For this review, take the finished solid that the model builds, in its own axes (mm). A direction names the side the tool comes from. Round coordinates to 2 decimals unless told otherwise and drop trailing zeros. Order: outer loops, then holes, each group sorted by start corner. A loop starts at its lowest first (then second) coordinate and runs counter-clockwise, first axis right, second up. Notation, with made-up numbers: M 3,36 L 16,36 A15 ccw 16,42 Z; hole C 17.5,86.25 d8. An arc over 180 degrees is marked long. Use a Markdown table: item, result.
from build123d import *

# Parameters (mm, degrees)
BOSS_EXTRUDE1_DEPTH = 1
BOSS_EXTRUDE2_START = 1
BOSS_EXTRUDE2_DEPTH = 1.6
BOSS_EXTRUDE3_START = 2.6
BOSS_EXTRUDE3_DEPTH = 1.3
BOSS_EXTRUDE4_START = 3.9
BOSS_EXTRUDE4_DEPTH = 1
FILLET1_R           = 1
CHAMFER1_SIZE       = 1.1


with BuildPart() as part:
    # Sketch1 → Boss-Extrude1 (new body)
    with BuildSketch(Plane(origin=(0, 0, 0), x_dir=(1, 0, 0), z_dir=(0, 1, 0))):
        with BuildLine():
            Line((-18.4, 13.7), (-18.4, 12.505918748))
            ThreePointArc((-18.4, 12.505918748), (-11.9, 4.9), (-18.4, -2.705918748))
            Line((-18.4, -2.705918748), (-18.4, -13.7))
            Line((-18.4, -13.7), (18.4, -13.7))
            Line((18.4, -13.7), (18.4, 13.7))
            Line((18.4, 13.7), (-18.4, 13.7))
        make_face()
        with BuildLine():
            ThreePointArc((-18.4, -2.705918748), (-11.9, 4.9), (-18.4, 12.505918748))
            Line((-18.4, 12.505918748), (-18.4, 10.472252686))
            ThreePointArc((-18.4, 10.472252686), (-13.9, 4.9), (-18.4, -0.672252686))
            Line((-18.4, -0.672252686), (-18.4, -2.705918748))
        make_face()
        with BuildLine():
            Line((19.6, 14.9), (-19.6, 14.9))
            Line((-19.6, 14.9), (-19.6, 12.6))
            ThreePointArc((-19.6, 12.6), (-18.998158808, 12.576443654), (-18.4, 12.505918748))
            Line((-18.4, 12.505918748), (-18.4, 13.7))
            Line((-18.4, 13.7), (18.4, 13.7))
            Line((18.4, 13.7), (18.4, -13.7))
            Line((18.4, -13.7), (-18.4, -13.7))
            Line((-18.4, -13.7), (-18.4, -2.705918748))
            ThreePointArc((-18.4, -2.705918748), (-18.998158808, -2.776443654), (-19.6, -2.8))
            Line((-19.6, -2.8), (-19.6, -14.9))
            Line((-19.6, -14.9), (19.6, -14.9))
            Line((19.6, -14.9), (19.6, 14.9))
        make_face()
        with BuildLine():
            ThreePointArc((-18.4, 12.505918748), (-18.998158808, 12.576443654), (-19.6, 12.6))
            Line((-19.6, 12.6), (-19.6, 10.6))
            ThreePointArc((-19.6, 10.6), (-18.996609708, 10.567973196), (-18.4, 10.472252686))
            Line((-18.4, 10.472252686), (-18.4, 12.505918748))
        make_face()
        with BuildLine():
            ThreePointArc((-18.4, -0.672252686), (-18.996609708, -0.767973196), (-19.6, -0.8))
            Line((-19.6, -0.8), (-19.6, -2.8))
            ThreePointArc((-19.6, -2.8), (-18.998158808, -2.776443654), (-18.4, -2.705918748))
            Line((-18.4, -2.705918748), (-18.4, -0.672252686))
        make_face()
    extrude(amount=BOSS_EXTRUDE1_DEPTH)

    # Sketch1<5> → Boss-Extrude2 (add)
    with BuildSketch(Plane(origin=(0, 0, 0), x_dir=(1, 0, 0), z_dir=(0, 1, 0)).offset(BOSS_EXTRUDE2_START)):
        with BuildLine():
            Line((-18.4, 13.7), (-18.4, 12.505918748))
            ThreePointArc((-18.4, 12.505918748), (-11.9, 4.9), (-18.4, -2.705918748))
            Line((-18.4, -2.705918748), (-18.4, -13.7))
            Line((-18.4, -13.7), (18.4, -13.7))
            Line((18.4, -13.7), (18.4, 13.7))
            Line((18.4, 13.7), (-18.4, 13.7))
        make_face()
        with BuildLine():
            ThreePointArc((-18.4, -2.705918748), (-11.9, 4.9), (-18.4, 12.505918748))
            Line((-18.4, 12.505918748), (-18.4, 10.472252686))
            ThreePointArc((-18.4, 10.472252686), (-13.9, 4.9), (-18.4, -0.672252686))
            Line((-18.4, -0.672252686), (-18.4, -2.705918748))
        make_face()
        with BuildLine():
            ThreePointArc((-18.4, 12.505918748), (-18.998158808, 12.576443654), (-19.6, 12.6))
            Line((-19.6, 12.6), (-19.6, 10.6))
            ThreePointArc((-19.6, 10.6), (-18.996609708, 10.567973196), (-18.4, 10.472252686))
            Line((-18.4, 10.472252686), (-18.4, 12.505918748))
        make_face()
        with BuildLine():
            ThreePointArc((-18.4, -0.672252686), (-18.996609708, -0.767973196), (-19.6, -0.8))
            Line((-19.6, -0.8), (-19.6, -2.8))
            ThreePointArc((-19.6, -2.8), (-18.998158808, -2.776443654), (-18.4, -2.705918748))
            Line((-18.4, -2.705918748), (-18.4, -0.672252686))
        make_face()
        with BuildLine():
            Line((19.6, 14.9), (-19.6, 14.9))
            Line((-19.6, 14.9), (-19.6, 12.6))
            ThreePointArc((-19.6, 12.6), (-18.998158808, 12.576443654), (-18.4, 12.505918748))
            Line((-18.4, 12.505918748), (-18.4, 13.7))
            Line((-18.4, 13.7), (18.4, 13.7))
            Line((18.4, 13.7), (18.4, -13.7))
            Line((18.4, -13.7), (-18.4, -13.7))
            Line((-18.4, -13.7), (-18.4, -2.705918748))
            ThreePointArc((-18.4, -2.705918748), (-18.998158808, -2.776443654), (-19.6, -2.8))
            Line((-19.6, -2.8), (-19.6, -14.9))
            Line((-19.6, -14.9), (19.6, -14.9))
            Line((19.6, -14.9), (19.6, 14.9))
        make_face()
    extrude(amount=BOSS_EXTRUDE2_DEPTH)

    # Sketch1<6> → Boss-Extrude3 (add)
    with BuildSketch(Plane(origin=(0, 0, 0), x_dir=(1, 0, 0), z_dir=(0, 1, 0)).offset(BOSS_EXTRUDE3_START)):
        with BuildLine():
            Line((-18.4, 13.7), (-18.4, 12.505918748))
            ThreePointArc((-18.4, 12.505918748), (-11.9, 4.9), (-18.4, -2.705918748))
            Line((-18.4, -2.705918748), (-18.4, -13.7))
            Line((-18.4, -13.7), (18.4, -13.7))
            Line((18.4, -13.7), (18.4, 13.7))
            Line((18.4, 13.7), (-18.4, 13.7))
        make_face()
        with BuildLine():
            ThreePointArc((-18.4, -2.705918748), (-11.9, 4.9), (-18.4, 12.505918748))
            Line((-18.4, 12.505918748), (-18.4, 10.472252686))
            ThreePointArc((-18.4, 10.472252686), (-13.9, 4.9), (-18.4, -0.672252686))
            Line((-18.4, -0.672252686), (-18.4, -2.705918748))
        make_face()
    extrude(amount=BOSS_EXTRUDE3_DEPTH)

    # Sketch1<8> → Boss-Extrude4 (add)
    with BuildSketch(Plane(origin=(0, 0, 0), x_dir=(1, 0, 0), z_dir=(0, 1, 0)).offset(BOSS_EXTRUDE4_START)):
        with BuildLine():
            ThreePointArc((-18.4, -2.705918748), (-11.9, 4.9), (-18.4, 12.505918748))
            Line((-18.4, 12.505918748), (-18.4, 10.472252686))
            ThreePointArc((-18.4, 10.472252686), (-13.9, 4.9), (-18.4, -0.672252686))
            Line((-18.4, -0.672252686), (-18.4, -2.705918748))
        make_face()
    extrude(amount=BOSS_EXTRUDE4_DEPTH)

    # Fillet1
    fillet1_edges = [part.edges().sort_by_distance(p)[0] for p in [
        (-11.9, 4.9, -4.9),
        (-18.4, 4.9, 1.689085717),
        (-18.4, 4.9, -11.489085717),
    ]]
    fillet(fillet1_edges, radius=FILLET1_R - 0.0001)  # a hair under: the kernel refuses the full size

    # Chamfer1
    chamfer1_edges = [part.edges().sort_by_distance(p)[0] for p in [
        (0, 0, 14.9),
        (-19.6, 0, 7.85),
        (-19.6, 0, -12.75),
        (0, 0, -14.9),
        (19.6, 0, 0),
    ]]
    chamfer(chamfer1_edges, length=CHAMFER1_SIZE)


solid = part.part
Q1. Add section D-D (y = 4.35). Write out the cut boundary in (x, z), then the cut area to 3 significant figures.
Determined:
| item | result |
|---|---|
| outline | M -18.29,-12.38 A7.59 ccw -18.29,2.58 L -18.29,0.65 A5.7 cw -18.29,-10.45 Z |
| area | 34.5 mm^2 |
Q2. Clearance check with flat-ended pins moving along their axes: pin 1 (13.5 mm diameter, centred on x = 7, z = -5.5, fed in from +Y); pin 2 (1 mm diameter, centred on x = -5, y = 3.5, fed in from -Z); pin 3 (1.4 mm diameter, centred on x = 9, y = 3.5, fed in from +Z). State where each tip first meets the part, or that it passes through.
Determined:
| item | result |
|---|---|
| pin 1 | stops at y = 3.9 |
| pin 2 | stops at z = -13.7 |
| pin 3 | stops at z = 13.7 |
Q3. Add section B-B (x = 5). Write out the cut boundary in (y, z).
Determined:
| item | result |
|---|---|
| outline | M 0,-13.8 L 1.1,-14.9 L 2.6,-14.9 L 2.6,-13.7 L 3.9,-13.7 L 3.9,13.7 L 2.6,13.7 L 2.6,14.9 L 1.1,14.9 L 0,13.8 Z |
Q4. Machinability: for faces 1 (the flat face through (0, 3, -13.7)), 2 (the flat face through (0, 3, 13.7)), 3 (the flat face through (-18.4, 3, 7)), 4 (the flat face through (19.1, 0.6, 0.2)), which of the approach directions +Z, -Z, +X, -X, +Y, -Y give a long, thin tool a straight path to every point of the face, cutting with its end or side? Answer none if there is none.
Determined:
| item | result |
|---|---|
| face 1 | -Z, +X, -X, +Y |
| face 2 | +Z, +X, -X, +Y |
| face 3 | +Z, -Z, -X, +Y |
| face 4 | +Z, -Z, +X, -Y |
Q5. Add section C-C (y = 1.6). Write out the cut boundary in (x, z).
Determined:
| item | result |
|---|---|
| outline | M -19.6,-14.9 L 19.6,-14.9 L 19.6,14.9 L -19.6,14.9 L -19.6,0.8 A5.7 cw -19.6,-10.6 Z |
Q6. Wall thickness on line 1 along Z through (x, y) = (13, 3.5); line 2 along Y through (x, z) = (5, -10.5); line 3 along X through (y, z) = (3.6, 2): over which ranges is each line inside the solid? List them lowest first. Write a range as [from, to].
Determined:
| item | result |
|---|---|
| line 1 | z = [-13.7, 13.7] |
| line 2 | y = [0, 3.9] |
| line 3 | x = [-18.4, 18.4] |
